```python
from build123d import *

# Parameters (mm, degrees)
SKETCH1_R           = 2.5
BOSS_EXTRUDE1_DEPTH = 8
CUT_EXTRUDE1_START  = 4
CUT_EXTRUDE1_DEPTH  = 4
FILLET1_R           = 5


with BuildPart() as part:
    # Sketch1 → Boss-Extrude1 (new body)
    with BuildSketch(Plane.XY):
        with BuildLine():
            ThreePointArc((9.097153376, 4.152324704), (7.50458322, 6.609177763), (5.268689672, 8.499465227))
            Line((5.268689672, 8.499465227), (4.99754882, -0.156543244))
            ThreePointArc((4.99754882, -0.156543244), (-0.780009037, -4.938783848), (-4.802546561, 1.391239206))
            Line((-4.802546561, 1.391239206), (-2.392849571, 9.709493855))
            ThreePointArc((-2.392849571, 9.709493855), (-6.876600935, 7.260327787), (-9.565391616, 2.916038962))
            ThreePointArc((-9.565391616, 2.916038962), (-1.474124119, -9.890751138), (10, 0))
            ThreePointArc((10, 0), (9.771681886, 2.124672473), (9.097153376, 4.152324704))
        make_face()
        with BuildLine():
            Line((4.99754882, -0.156543244), (5.268689672, 8.499465227))
            ThreePointArc((5.268689672, 8.499465227), (1.560018074, 9.877567697), (-2.392849571, 9.709493855))
            Line((-2.392849571, 9.709493855), (-4.802546561, 1.391239206))
            ThreePointArc((-4.802546561, 1.391239206), (0.702590633, 4.95039053), (5, 0))
            ThreePointArc((5, 0), (4.999387168, -0.078281216), (4.99754882, -0.156543244))
        make_face()
        with BuildLine():
            ThreePointArc((5.620036149, 19.755135394), (5.619729732, 19.715994786), (5.618810559, 19.676863772))
            Line((5.618810559, 19.676863772), (5.268689672, 8.499465227))
            ThreePointArc((5.268689672, 8.499465227), (7.50458322, 6.609177763), (9.097153376, 4.152324704))
            Line((9.097153376, 4.152324704), (12.147237195, 8.825258116))
            ThreePointArc((12.147237195, 8.825258116), (13.442669974, 22.004389763), (18.247609257, 34.344576778))
            Line((18.247609257, 34.344576778), (0, 34.293094604))
            Line((0, 34.293094604), (-9.565391616, 2.916038962))
            ThreePointArc((-9.565391616, 2.916038962), (-6.876600935, 7.260327787), (-2.392849571, 9.709493855))
            Line((-2.392849571, 9.709493855), (0.718762868, 20.450754997))
            ThreePointArc((0.718762868, 20.450754997), (3.471331465, 22.230330659), (5.620036149, 19.755135394))
        make_face()
        with BuildLine():
            Line((5.268689672, 8.499465227), (5.618810559, 19.676863772))
            ThreePointArc((5.618810559, 19.676863772), (2.73003163, 17.28574347), (0.718762868, 20.450754997))
            Line((0.718762868, 20.450754997), (-2.392849571, 9.709493855))
            ThreePointArc((-2.392849571, 9.709493855), (1.560018074, 9.877567697), (5.268689672, 8.499465227))
        make_face()
        with Locations((3.120036149, 19.755135394)):
            Circle(SKETCH1_R)
    extrude(amount=BOSS_EXTRUDE1_DEPTH)

    # Sketch1<3> → Cut-Extrude1 (cut)
    with BuildSketch(Plane.XY.offset(CUT_EXTRUDE1_START)):
        with BuildLine():
            ThreePointArc((5.618810559, 19.676863772), (3.510040667, 22.224527318), (0.718762868, 20.450754997))
            Line((0.718762868, 20.450754997), (-4.802546561, 1.391239206))
            ThreePointArc((-4.802546561, 1.391239206), (0.780009037, 4.938783848), (4.99754882, -0.156543244))
            Line((4.99754882, -0.156543244), (5.618810559, 19.676863772))
        make_face()
    extrude(amount=CUT_EXTRUDE1_DEPTH, mode=Mode.SUBTRACT)

    # Fillet1
    fillet1_edges = [part.edges().sort_by_distance(p)[0] for p in [
        (12.147237195, 8.825258116, 4),
    ]]
    fillet(fillet1_edges, radius=FILLET1_R)


solid = part.part
```
Work out the finished part from the listing and answer in its coordinate system (mm). A direction names the side the tool comes from. Coordinates: 2 decimals unless noted, no trailing zeros. Write each loop counter-clockwise with the first axis right and the second up, starting at its lowest first coordinate (ties: lowest second). Pieces come first, ordered by that corner, then holes.
Q1. Each of these flat-tipped pins is pushed along its axis until it touches: pin 1 Ø1 at (y, z) = (19, 1.5) entering from -X; pin 2 Ø1 at (x, z) = (-1, 4) entering from -Y. Where does it stop, or does it pass through?
Q2. A cutting plane is placed at A-A, the plane x = -3.5. Give the vertices of the cut face in (y, z).
Q3. A cutting plane is placed at D-D, the plane z = 1. Give the vertices of the cut face in (x, y).
Q4. Find the intervals of material crossed by line 1 (X direction, y = 0, z = 5.5); line 2 (Z direction, x = 5, y = 10); line 3 (X direction, y = 3, z = 4.5), in increasing order.
Q5. A cutting plane is placed at B-B, the plane y = 12.5. Give the vertices of the cut face in (x, z).
Q6. A cutting plane is placed at C-C, the plane z = 4.5. Give the vertices of the cut face in (x, y).
Q7. Which of the six approach directions +Z, -Z, +X, -X, +Y, -Y give full straight-line access (tool end or side, diameter ignored) to faces 1 (the face through (10.183, 5.816, 3.944)), 2 (the face through (3, 11, 4)), 3 (the face through (4, 12, 0))?
Findings below:
1. pin 1: stops at x = -4.81
1. pin 2: stops at y = -9.99
2. outline: (-9.37, 0) - (-3.57, 0) - (-3.57, 8) - (-9.37, 8) - close; (3.57, 0) - (22.81, 0) - (22.81, 8) - (5.89, 8) - (5.89, 4) - (3.57, 4) - close
3. outline: (-9.57, 2.92) arc R10 ccw (long way) to (9.1, 4.15) - (11.3, 7.53) arc R5 ccw to (12.11, 10.3) arc R48.6 cw to (18.25, 34.34) - (0, 34.29) - close; hole (5, -0.16) arc R5 ccw to (5, 0) arc R5 ccw (long way) to start
4. line 1: x = -10 to -5, 5 to 10
4. line 2: z = 0 to 4
4. line 3: x = -9.54 to -4.34, 5.1 to 9.54
5. outline: (-6.64, 0) - (12.14, 0) - (12.14, 8) - (5.39, 8) - (5.39, 4) - (-1.58, 4) - (-1.58, 8) - (-6.64, 8) - close
6. outline: (-9.57, 2.92) arc R10 ccw (long way) to (9.1, 4.15) - (11.3, 7.53) arc R5 ccw to (12.11, 10.3) arc R48.6 cw to (18.25, 34.34) - (0, 34.29) - close; hole (-4.8, 1.39) arc R5 ccw (long way) to (5, -0.16) - (5.62, 19.68) arc R2.5 ccw to (0.72, 20.45) - close
7. face 1: +Z, -Z, +X
7. face 2: +Z
7. face 3: -Z, +X, -X, +Y, -Y
